CAD build for the part. Positions are in the model's coordinates, mm. Give positions to 0.01 mm unless a question says otherwise; leave off trailing zeros. Order: outer loops, then holes, each group sorted by start corner. A loop starts at its lowest first (then second) coordinate and runs counter-clockwise, first axis right, second up.
Item 1: Wall check: L1, parallel to Y at x = -256, z = 50.5; L2, parallel to Y at x = 268, z = 14.5; L3, parallel to X at y = 327.5, z = 47.5. Give the ranges that are in metal, low to high.
Item 2: Band-saw the part on B-B on y = 178. Give the cut face in (x, z).
Item 3: Flat gauge pins, fed straight in: P1, Ø12, axis at y = 560.5, z = 12, coming from the -X side; P2, Ø4, axis at x = 80, z = 23.5, coming from the +Y side; P3, Ø6, axis at x = 318.5, z = 8, coming from the +Y side. Where does each tip first touch, or does it go through?
Item 4: Band-saw the part on A-A on z = 14.5. Give the cut face in (x, y).
Item 5: Two-plate mould, pull along Y, no slides. Class faces 1 (the cylindrical face through (218.02, 872.21, 27.12)), 2 (the flat face through (436, 418, 27)), 3 (the flat face through (354.91, 886.55, 27.12)): released by +Y, released by -Y, zero draft, split by the parting line, or undercut.
Item 6: Band-saw the part on C-C on x = -207.5. Give the cut face in (y, z), plus the area to 3 significant figures.
```python
from build123d import *

# Parameters (mm, degrees)
SKETCH1_R           = 25
SKETCH1_R_2         = 15
BOSS_EXTRUDE1_DEPTH = 55


with BuildPart() as part:
    # Sketch1 → Boss-Extrude1 (new body)
    with BuildSketch(Plane.XY):
        with BuildLine():
            Line((0, 0), (436, 0))
            Line((436, 0), (436, 847))
            Line((436, 847), (271.520689527, 927.221919862))
            ThreePointArc((271.520689527, 927.221919862), (202.977427959, 927.978702538), (159.009788885, 875.389747989))
            ThreePointArc((159.009788885, 875.389747989), (44.140964675, 543.56321378), (-252.456286899, 355.590433997))
            ThreePointArc((-252.456286899, 355.590433997), (-283.190978989, 339.913558022), (-306.768623817, 314.724663594))
            Line((-306.768623817, 314.724663594), (-372.987704373, 236.21505403))
            ThreePointArc((-372.987704373, 236.21505403), (-155.534588664, 166.992745943), (0, 0))
        make_face()
        with Locations((236.450997784, 855.318396158)):
            Circle(SKETCH1_R, mode=Mode.SUBTRACT)
        with Locations((-242.894848687, 286.21505403)):
            Circle(SKETCH1_R_2, mode=Mode.SUBTRACT)
    extrude(amount=BOSS_EXTRUDE1_DEPTH)


solid = part.part
```
The answers:
1. L1: y = 214.39 to 278.92, 293.51 to 354.43
1. L2: y = 0 to 928.83
1. L3: x = -296.85 to 436
2. outline: (-173.86, 0) - (436, 0) - (436, 55) - (-173.86, 55) - close
3. P1: stops at x = 52.57
3. P2: stops at y = 598.06
3. P3: stops at y = 905.77
4. outline: (-372.99, 236.22) arc R450 cw to (0, 0) - (436, 0) - (436, 847) - (271.52, 927.22) arc R80 ccw to (159.01, 875.39) arc R532 cw to (-252.46, 355.59) arc R100 ccw to (-306.77, 314.72) - close; hole circle Ø30 at (-242.89, 286.22); hole circle Ø50 at (236.45, 855.32)
5. face 1: undercut
5. face 2: zero draft
5. face 3: released by +Y
6. outline: (195.3, 0) - (368.15, 0) - (368.15, 55) - (195.3, 55) - close
6. area: 9,510 mm2
